```python
from build123d import *

# Parameters (mm, degrees)
F1_DEPTH  = 16
F6_DEPTH  = 6
F7_DEPTH  = 3
F8_DEPTH  = 3
F9_R      = 4
F12_DEPTH = 25
F11_R     = 3
F13_DEPTH = 50
F10_R     = 3
F14_DEPTH = 50


with BuildPart() as f1:
    # F0 (on Front) → F1 (new body)
    with BuildSketch(Plane.XZ):
        Polygon((0, 0), (0, 72), (-3, 72), (-3, 1.127205), (-10, -6.872795), (-10, -31.291796), (-14, -39.291796), (-14, -72.708204), (-10, -80.708204), (-10, -86), (-7, -86), (-7, -80), (-11, -72), (-11, -40), (-7, -32), (-7, -8), align=None)
    extrude(amount=F1_DEPTH)

    # F2: F1 across plane


with BuildPart() as f1_1:
    add(f1.part)
    add(f1.part.mirror(Plane.YZ))

    # F3 (on face) → F6 (join)
    with BuildSketch(Plane.YZ.offset(3)):
        with BuildLine():
            Line((-16, 72), (0, 72))
            ThreePointArc((0, 72), (-8, 80), (-16, 72))
        make_face()
    extrude(amount=-F6_DEPTH)

    # F5 (on face) → F7 (join)
    with BuildSketch(Plane(origin=(-10, 0, 0), x_dir=(0, -1, 0), z_dir=(-1, 0, 0))):
        with BuildLine():
            Line((16, -86), (0, -86))
            ThreePointArc((0, -86), (8, -94), (16, -86))
        make_face()
    extrude(amount=-F7_DEPTH)

    # F4 (on face) → F8 (join)
    with BuildSketch(Plane.YZ.offset(10)):
        with BuildLine():
            Line((0, -86), (-16, -86))
            ThreePointArc((-16, -86), (-8, -94), (0, -86))
        make_face()
    extrude(amount=-F8_DEPTH)

    # F9 (on face) → F12 (cut)
    with BuildSketch(Plane.YZ.offset(3)):
        with Locations((-8, 72)):
            Circle(F9_R)
    extrude(amount=-F12_DEPTH, mode=Mode.SUBTRACT)

    # F11 (on face) → F13 (cut)
    with BuildSketch(Plane.YZ.offset(10)):
        with Locations((-8, -19.082295)):
            Circle(F11_R)
    extrude(amount=-F13_DEPTH, mode=Mode.SUBTRACT)

    # F10 (on face) → F14 (cut)
    with BuildSketch(Plane.YZ.offset(10)):
        with Locations((-8, -86)):
            Circle(F10_R)
    extrude(amount=-F14_DEPTH, mode=Mode.SUBTRACT)


solid = f1_1.part
```
The model under review builds one solid part; all positions refer to its coordinate system, in mm. A direction names the side the tool comes from. Give positions to 0.01 mm unless a question says otherwise; leave off trailing zeros. Write each loop counter-clockwise with the first axis right and the second up, starting at its lowest first coordinate (ties: lowest second). Pieces come first, ordered by that corner, then holes. Notation, with made-up numbers: M 44,17.25 L 57,17.25 A18 ccw 57,50.25 Z; hole C -13.75,-7.5 d4. An arc over 180 degrees is marked long. Answer in a Markdown table with one row per item.
Item 1: For line 1 along X through (y, z) = (-2.25, -53); line 2 along Z through (x, y) = (-8.75, -8); line 3 along Z through (x, y) = (-1.75, -10.5), list the stretches that pass through material, from the lowest coordinate up.
Check sheet entries:
| item | result |
|---|---|
| line 1 | -14 to -11, 11 to 14 |
| line 2 | -94 to -89, -83 to -76.5, -35.5 to -22.08, -16.08 to -5.44 |
| line 3 | -2 to 68.88, 75.12 to 79.6 |
Item 2: Tool access review of faces 5 (the face through (9, -8, -76)), 6 (the face through (-7, -8, -23)), 7 (the face through (10, -6, -89)): name each direction out of +Z, -Z, +X, -X, +Y, -Y from which nothing blocks a thin tool from reaching the whole face with its end or side.
Check sheet entries:
| item | result |
|---|---|
| face 5 | +Y, -Y |
| face 6 | -Z, +Y, -Y |
| face 7 | -Z, +X, +Y, -Y |
Item 3: Add section C-C on z = -3. Give the boundary of the cut face in (x, y) (3 decimals).
Check sheet entries:
| item | result |
|---|---|
| outline | M -6.611,-16 L -2.625,-16 L -2.625,0 L -6.611,0 Z; M 2.625,-16 L 6.611,-16 L 6.611,0 L 2.625,0 Z |
Item 4: For P1, Ø8, axis at y = -11.5, z = -25, coming from the -X side; P2, Ø5, axis at y = -9.5, z = 32, coming from the -X side; P3, Ø6, axis at x = 7, y = -10, coming from the +Z side, all flat-tipped, find the tip position at first contact; note any pin that passes through.
Check sheet entries:
| item | result |
|---|---|
| P1 | x = -10 |
| P2 | x = -3 |
| P3 | z = -0.02 |
Item 5: Add section D-D on z = 66. Give the boundary of the cut face in (x, y), plus the area to 3 significant figures.
Check sheet entries:
| item | result |
|---|---|
| outline | M -3,-16 L 3,-16 L 3,0 L -3,0 Z |
| area | 96.0 mm2 |
Item 6: Add section B-B on y = -8. State how many separate pieces and enclosed holes the cut face has, plus the area to 3 significant figures.
Check sheet entries:
| item | result |
|---|---|
| separate pieces | 6 |
| enclosed holes | 0 |
| area | 951 mm2 |
Item 7: Draft analysis for pull direction X (two halves, no side actions). For faces 1 (the face through (3, -8, 41)), 2 (the face through (-11, -8, -56)), 3 (the face through (-9, -8, -94)), 4 (the face through (-12.03, -7.89, -76.65)), state which applies: +X half, -X half, draft (parallel to the pull), parting line (faces both ways), or undercut.
Check sheet entries:
| item | result |
|---|---|
| face 1 | +X half |
| face 2 | undercut |
| face 3 | draft |
| face 4 | -X half |
Item 8: Add section A-A on z = -61.5. Give the boundary of the cut face in (x, y), plus the area to 3 significant figures.
Check sheet entries:
| item | result |
|---|---|
| outline | M -14,-16 L -11,-16 L -11,0 L -14,0 Z; M 11,-16 L 14,-16 L 14,0 L 11,0 Z |
| area | 96.0 mm2 |
